Autodesk Inventor part; units mm, degrees
ref_plane "YZ Plane" through (0, 0, 0) normal (1, 0, 0) x (0, 1, 0)
ref_plane "XZ Plane" through (0, 0, 0) normal (0, 1, 0) x (-1, 0, 0)
ref_plane "XY Plane" through (0, 0, 0) normal (0, 0, 1) x (1, 0, 0)
sketch "Schizzo1" plane through (0, 0, 0) normal (0, 0, 1) x (1, 0, 0)
  arc A0 (36.9231, 17.4874) -> (37.9231, 18.4874) centre (36.9231, 18.4874) ccw
  line L0 (27.9231, 37.356) -> (27.9231, 17.6188) construction
  line L1 (36.9231, 17.4874) -> (30.9231, 17.4874)
  line L2 (30.9231, 19.4874) -> (33.9231, 19.4874)
  line L3 (30.9231, 19.4874) -> (30.9231, 17.4874)
  line L4 (33.9231, 19.4874) -> (33.9231, 20.5217)
  line L5 (35.9231, 21.4874) -> (35.1213, 21.4874)
  line L6 (33.9231, 20.5217) -> (30.9273, 23.4874)
  line L7 (31.958, 23.6188) -> (32.4267, 23.6188) construction
  line L8 (35.1213, 21.4874) -> (31.9231, 24.6188)
  line L9 (27.9231, 28.7445) -> (27.9203, 28.7473)
  line L10 (27.9231, 27.4874) -> (16.785, 27.4874) construction
  line L11 (35.9231, 21.4874) -> (35.9231, 24.4874)
  line L12 (35.9231, 24.4874) -> (37.9231, 24.4874)
  line L13 (37.9231, 24.4874) -> (37.9231, 18.4874)
  line L14 (0.5417, 54.5893) -> (0.5417, -0.7152) construction
  arc A1 (17.9231, 18.4874) -> (18.9231, 17.4874) centre (18.9231, 18.4874) ccw
  line L15 (18.9231, 17.4874) -> (24.9231, 17.4874)
  line L16 (24.9231, 19.4874) -> (21.9231, 19.4874)
  line L17 (24.9231, 19.4874) -> (24.9231, 17.4874)
  line L18 (21.9231, 19.4874) -> (21.9231, 20.5217)
  line L19 (19.9231, 21.4874) -> (20.725, 21.4874)
  line L20 (21.9231, 20.5217) -> (24.919, 23.4874)
  line L21 (23.958, 23.6188) -> (23.9231, 23.6188) construction
  line L22 (19.9231, 21.4874) -> (19.9231, 24.4874)
  line L23 (19.9231, 24.4874) -> (17.9231, 24.4874)
  line L24 (17.9231, 24.4874) -> (17.9231, 18.4874)
  line L25 (33.8225, 24.3529) -> (33.8225, 24.4874)
  arc A2 (37.9231, 36.4874) -> (36.9231, 37.4874) centre (36.9231, 36.4874) ccw
  line L26 (36.9231, 37.4874) -> (30.9231, 37.4874)
  line L27 (30.9231, 35.4874) -> (33.9231, 35.4874)
  line L28 (30.9231, 35.4874) -> (30.9231, 37.4874)
  line L29 (33.9231, 35.4874) -> (33.9231, 34.4531)
  line L30 (35.9231, 33.4874) -> (35.1213, 33.4874)
  line L31 (33.9231, 34.4531) -> (30.9273, 31.4874)
  line L32 (31.958, 31.356) -> (32.4267, 31.356) construction
  line L33 (35.1213, 33.4874) -> (31.9231, 30.356)
  line L34 (35.9231, 33.4874) -> (35.9231, 30.4874)
  line L35 (35.9231, 30.4874) -> (37.9231, 30.4874)
  line L36 (37.9231, 30.4874) -> (37.9231, 36.4874)
  arc A3 (18.9231, 37.4874) -> (17.9231, 36.4874) centre (18.9231, 36.4874) ccw
  line L37 (19.9231, 30.4874) -> (17.9231, 30.4874)
  line L38 (19.9231, 33.4874) -> (20.725, 33.4874)
  line L39 (19.9231, 33.4874) -> (19.9231, 30.4874)
  line L40 (21.9231, 34.4531) -> (24.919, 31.4874)
  line L41 (24.9231, 35.4874) -> (21.9231, 35.4874)
  line L42 (21.9231, 35.4874) -> (21.9231, 34.4531)
  line L43 (24.9231, 35.4874) -> (24.9231, 37.4874)
  line L44 (18.9231, 37.4874) -> (24.9231, 37.4874)
  line L45 (17.9231, 30.4874) -> (17.9231, 36.4874)
  line L46 (33.8225, 30.6219) -> (33.8225, 30.4874)
  line L47 (30.9273, 23.4874) -> (24.919, 23.4874)
  line L48 (23.9231, 24.549) -> (23.9231, 30.4259)
  line L49 (24.919, 31.4874) -> (30.9273, 31.4874)
  line L50 (31.9231, 30.356) -> (31.9231, 24.6188)
  line L51 (23.9231, 24.549) -> (20.725, 21.4874)
  line L52 (23.9231, 30.4259) -> (20.725, 33.4874)
  circle A4 centre (27.9231, 27.4874) radius 2.1
  point P0 (0, 0)
  point P1 (17.9231, 17.6188)
  point P2 (22.0237, 24.3529)
  point P3 (24.8821, 25.7341)
  point P4 (23.4196, 23.6188)
  point P5 (17.9231, 37.356)
  point P6 (22.0237, 30.6219)
  point P7 (24.8821, 29.2408)
  point P8 (27.958, 27.4874)
  dimension "d104" = 20
  dimension "d111" = 8
  dimension "d112" = 4.2
  dimension "d115" = 20
  dimension "d116" = 6
  dimension "d117" = 4
  dimension "d118" = 1
  dimension "d119" = 12
  dimension "d129" = 6
  dimension "d130" = 6
  dimension "d131" = 6
  dimension "d132" = 2
  dimension "d133" = 2
  dimension "d134" = 2
  dimension "d135" = 2
  dimension "d136" = 12
  dimension "d137" = 12
  dimension "d146" = 8
extrude "Estrusione1" add sketch "Schizzo1" along normal blind 20
properties part number "Aluminium profile 20x20 6mm slot"
Geometry: final body of the model. Coordinates: model frame, mm. A direction names the side the tool comes from. Round coordinates to 2 decimals unless told otherwise and drop trailing zeros. Order: outer loops, then holes, each group sorted by start corner. A loop starts at its lowest first (then second) coordinate and runs counter-clockwise, first axis right, second up. Notation, with made-up numbers: (-29.75, -3) - (-23.75, -3) arc R25 ccw to (-23.75, 30) - close; hole circle Ø4 at (-14.75, 81.25). An arc over 180 degrees is marked (long way). Write item = value, one per line. Start each with the question number.
Q1. Cut plane B-B on y = 28. Return the cut outline in (x, z).
Q2. Pull-direction query (Y, two-part tool) for faces 4 (the cylindrical face through (37.64, 17.79, 9.86)), 5 (the flat face through (28, 31.487, 10)), 6 (the flat face through (23, 19.487, 10)), 7 (the flat face through (25.6, 27.6, 20)); classes: +Y half, -Y half, draft (parallel to the pull), parting line (faces both ways), or undercut.
Q3. Ray query, line 1 (Y direction, x = 33.25, z = 11); line 2 (Y direction, x = 23.5, z = 10.25); line 3 (Y direction, x = 19.75, z = 18.75). Return the intervals inside material, ascending. Write a range as from..to.
Q4. Cut plane A-A on x = 26.25. Return the cut outline in (y, z), and give its area (3 significant figures).
Q5. Access query for faces 1 (the flat face through (19, 24.487, 10)), 2 (the flat face through (22.346, 31.935, 9.86)), 3 (the flat face through (30.923, 19, 10)). Directions: +Z, -Z, +X, -X, +Y, -Y. A direction counts if a zero-diameter tool reaches every point of the face in a straight line with its end or side. Return the directions, or none.
Q6. Pin query (flat end, axial travel): pin 1 (1.8 mm diameter, centred on y = 28, z = 9.5, fed in from -X); pin 2 (1.8 mm diameter, centred on x = 27.5, z = 10.5, fed in from -Y). Return the tip coordinate at first contact, or that it passes through.
Q7. Cut plane D-D on x = 23. Return the cut outline in (y, z).
Q8. Cut plane C-C on y = 24. Return the cut outline in (x, z).
Outcome:
q1.outline = (23.92, 0) - (25.89, 0) - (25.89, 20) - (23.92, 20) - close; (29.96, 0) - (31.92, 0) - (31.92, 20) - (29.96, 20) - close
q2.face_4 = -Y half
q2.face_5 = +Y half
q2.face_6 = undercut
q2.face_7 = draft
q3.line_1 = 17.49..19.49, 21.19..23.32, 31.66..33.79, 35.49..37.49
q3.line_2 = 17.49..19.49, 22.08..24.14, 30.83..32.89, 35.49..37.49
q3.line_3 = 17.49..24.49, 30.49..37.49
q4.outline = (23.49, 0) - (26.22, 0) - (26.22, 20) - (23.49, 20) - close; (28.76, 0) - (31.49, 0) - (31.49, 20) - (28.76, 20) - close
q4.area = 109 mm^2
q5.face_1 = +Z, -Z, -X
q5.face_2 = +Z, -Z
q5.face_3 = +Z, -Z, -Y
q6.pin_1 = 23.92
q6.pin_2 = 23.49
q7.outline = (17.49, 0) - (19.49, 0) - (19.49, 20) - (17.49, 20) - close; (21.59, 0) - (23.67, 0) - (23.67, 20) - (21.59, 20) - close; (31.31, 0) - (33.39, 0) - (33.39, 20) - (31.31, 20) - close; (35.49, 0) - (37.49, 0) - (37.49, 20) - (35.49, 20) - close
q8.outline = (17.92, 0) - (19.92, 0) - (19.92, 20) - (17.92, 20) - close; (23.35, 0) - (32.56, 0) - (32.56, 20) - (23.35, 20) - close; (35.92, 0) - (37.92, 0) - (37.92, 20) - (35.92, 20) - close
